Geometry: final body of the model. Coordinates: model frame, mm. Give positions to 0.01 mm unless a question says otherwise; leave off trailing zeros. Order: outer loops, then holes, each group sorted by start corner. A loop starts at its lowest first (then second) coordinate and runs counter-clockwise, first axis right, second up. Notation, with made-up numbers: (64.5, 50.25) - (108.5, 50.25) arc R6 ccw to (108.5, 59.25) - close; hole circle Ø10 at (72, 3.5). An arc over 180 degrees is marked (long way). One line per item, written item: value.
```python
from build123d import *

# Parameters (mm, degrees)
F0_R     = 11.627364
F0_R_2   = 5.06648
F1_DEPTH = 2.032
F2_R     = 1.651
F3_SIZE  = 0.254
F4_SIZE  = 0.254


with BuildPart() as f1:
    # F0 (on Top) → F1 (new body)
    with BuildSketch(Plane.XY):
        Circle(F0_R)
        Circle(F0_R_2, mode=Mode.SUBTRACT)
    extrude(amount=F1_DEPTH)

    # F2
    f2_edges = [f1.edges().sort_by_distance(p)[0] for p in [
        (-11.627364, 0, 2.032),
    ]]
    fillet(f2_edges, radius=F2_R)

    # F3
    f3_edges = [f1.edges().sort_by_distance(p)[0] for p in [
        (-5.06648, 0, 2.032),
    ]]
    chamfer(f3_edges, length=F3_SIZE)

    # F4
    f4_edges = [f1.edges().sort_by_distance(p)[0] for p in [
        (-5.06648, 0, 0),
    ]]
    chamfer(f4_edges, length=F4_SIZE)


solid = f1.part
```
1) Section C-C, the plane z = 1.15. Return loops of the section in (x, y), then the cut area to 3 significant figures.
Answers below:
outline: circle Ø22.87 at (0, 0); hole circle Ø10.13 at (0, 0)
area: 330 mm^2
2) Material intervals for line 1 along X through (y, z) = (2.75, 0.15); line 2 along Y through (x, z) = (0, 1.5); line 3 along Y through (x, z) = (-3.25, 0.1), sorted ascending.
Answers below:
line 1: -11.3 to -4.38, 4.38 to 11.3
line 2: -11.19 to -5.07, 5.07 to 11.19
line 3: -11.16 to -4.09, 4.09 to 11.16
3) Mould query, pull axis X, two halves, no side actions, for faces 1 (the face through (4, -4, 2.032)), 2 (the face through (-1.51, 11.53, 0.19)), 3 (the face through (4.833, 1.522, 1.005)). Classes: released by +X, released by -X, zero draft, split by the parting line, or undercut.
Answers below:
face 1: zero draft
face 2: split by the parting line
face 3: undercut
4) Section A-A, the plane y = 0. Return loops of the section in (x, z).
Answers below:
outline: (-11.63, 0) - (-5.32, 0) - (-5.07, 0.25) - (-5.07, 1.78) - (-5.32, 2.03) - (-9.98, 2.03) arc R1.65 ccw to (-11.63, 0.38) - close; (5.07, 0.25) - (5.32, 0) - (11.63, 0) - (11.63, 0.38) arc R1.65 ccw to (9.98, 2.03) - (5.32, 2.03) - (5.07, 1.78) - close
